Source: CAD feature listing. Evaluate the final solid. Frame: model axes, mm. A direction names the side the tool comes from. Round coordinates to 2 decimals unless told otherwise and drop trailing zeros. Loops run counter-clockwise (first coordinate to the right, second up) from the corner with the lowest first, then second, coordinate; pieces in that order, holes last. Notation, with made-up numbers: (49.25, 33.5) -> (105.25, 33.5) arc R23 ccw to (105.25, 52.5) -> close; hole circle Ø1 at (73, 71). An arc over 180 degrees is marked (long way). Write item = value, one per line.
from build123d import *

# Parameters (mm, degrees)
SKETCH_1_R          = 15.915
EXTRUDE_1_DEPTH     = 11
SKETCH_2_R          = 17
EXTRUDE_2_DEPTH     = 2
EXTRUDE_START       = 2
SKETCH_3_R          = 17
EXTRUDE_3_DEPTH     = 2
SKETCH_4_R          = 9.5
SKETCH_4_R_2        = 7.5
CUT_EXTRUDE_1_DEPTH = 0.5
SKETCH_4_3_R        = 7.5
SKETCH_4_3_R_2      = 5
CUT_EXTRUDE_2_DEPTH = 1.5
SKETCH_4_4_R        = 5
SKETCH_4_4_R_2      = 4
CUT_EXTRUDE_3_DEPTH = 0.5
SKETCH_4_5_R        = 4
CUT_EXTRUDE_4_DEPTH = 29.337254631
CUT_EXTRUDE_START   = -0.5
SKETCH_6_R          = 9.5
SKETCH_6_R_2        = 7.5
CUT_EXTRUDE_5_DEPTH = 0.5
CUT_EXTRUDE_START_2 = -1.5
SKETCH_6_3_R        = 7.5
SKETCH_6_3_R_2      = 5
CUT_EXTRUDE_6_DEPTH = 1.5
SKETCH_6_5_R        = 5
SKETCH_6_5_R_2      = 4
CUT_EXTRUDE_7_DEPTH = 0.5


with BuildPart() as part:
    # Sketch 1 → Extrude 1 (new body)
    with BuildSketch(Plane(origin=(0, 0, 0), x_dir=(1, 0, 0), z_dir=(0, 1, 0))):
        with Locations(Location((0, 0, 0), (0, 0, 270))):
            Circle(SKETCH_1_R)
    extrude(amount=EXTRUDE_1_DEPTH)

    # Sketch 2 → Extrude 2 (add)
    with BuildSketch(Plane(origin=(0, 11, 0), x_dir=(1, 0, 0), z_dir=(0, 1, 0))):
        with Locations(Location((0, 0, 0), (0, 0, 270))):
            Circle(SKETCH_2_R)
    extrude(amount=EXTRUDE_2_DEPTH)

    # Sketch 3 → Extrude 3 (add)
    with BuildSketch(Plane.XZ.offset(EXTRUDE_START)):
        with Locations(Location((0, 0, 0), (0, 0, 90))):
            Circle(SKETCH_3_R)
    extrude(amount=-EXTRUDE_3_DEPTH)

    # Sketch 4 → Cut-Extrude 1 (cut)
    with BuildSketch(Plane.XZ.offset(2)):
        with Locations(Location((0, 0, 0), (0, 0, 270))):
            Circle(SKETCH_4_R)
        with Locations(Location((0, 0, 0), (0, 0, 270))):
            Circle(SKETCH_4_R_2, mode=Mode.SUBTRACT)
    extrude(amount=-CUT_EXTRUDE_1_DEPTH, mode=Mode.SUBTRACT)

    # Sketch 4_3 → Cut-Extrude 2 (cut)
    with BuildSketch(Plane.XZ.offset(2)):
        with Locations(Location((0, 0, 0), (0, 0, 270))):
            Circle(SKETCH_4_3_R)
        with Locations(Location((0, 0, 0), (0, 0, 270))):
            Circle(SKETCH_4_3_R_2, mode=Mode.SUBTRACT)
    extrude(amount=-CUT_EXTRUDE_2_DEPTH, mode=Mode.SUBTRACT)

    # Sketch 4_4 → Cut-Extrude 3 (cut)
    with BuildSketch(Plane.XZ.offset(2)):
        with Locations(Location((0, 0, 0), (0, 0, 270))):
            Circle(SKETCH_4_4_R)
        with Locations(Location((0, 0, 0), (0, 0, 270))):
            Circle(SKETCH_4_4_R_2, mode=Mode.SUBTRACT)
    extrude(amount=-CUT_EXTRUDE_3_DEPTH, mode=Mode.SUBTRACT)

    # Sketch 4_5 → Cut-Extrude 4 (cut, through all)
    with BuildSketch(Plane.XZ.offset(2)):
        with Locations(Location((0, 0, 0), (0, 0, 270))):
            Circle(SKETCH_4_5_R)
    extrude(amount=-CUT_EXTRUDE_4_DEPTH, mode=Mode.SUBTRACT)

    # Sketch 6 → Cut-Extrude 5 (cut)
    with BuildSketch(Plane(origin=(0, 13, 0), x_dir=(1, 0, 0), z_dir=(0, 1, 0)).offset(CUT_EXTRUDE_START)):
        with Locations(Location((0, 0, 0), (0, 0, 90))):
            Circle(SKETCH_6_R)
        with Locations(Location((0, 0, 0), (0, 0, 90))):
            Circle(SKETCH_6_R_2, mode=Mode.SUBTRACT)
    extrude(amount=CUT_EXTRUDE_5_DEPTH, mode=Mode.SUBTRACT)

    # Sketch 6_3 → Cut-Extrude 6 (cut)
    with BuildSketch(Plane(origin=(0, 13, 0), x_dir=(1, 0, 0), z_dir=(0, 1, 0)).offset(CUT_EXTRUDE_START_2)):
        with Locations(Location((0, 0, 0), (0, 0, 90))):
            Circle(SKETCH_6_3_R)
        with Locations(Location((0, 0, 0), (0, 0, 90))):
            Circle(SKETCH_6_3_R_2, mode=Mode.SUBTRACT)
    extrude(amount=CUT_EXTRUDE_6_DEPTH, mode=Mode.SUBTRACT)

    # Sketch 6_5 → Cut-Extrude 7 (cut)
    with BuildSketch(Plane(origin=(0, 13, 0), x_dir=(1, 0, 0), z_dir=(0, 1, 0)).offset(CUT_EXTRUDE_START)):
        with Locations(Location((0, 0, 0), (0, 0, 270))):
            Circle(SKETCH_6_5_R)
        with Locations(Location((0, 0, 0), (0, 0, 90))):
            Circle(SKETCH_6_5_R_2, mode=Mode.SUBTRACT)
    extrude(amount=CUT_EXTRUDE_7_DEPTH, mode=Mode.SUBTRACT)


solid = part.part
1. Line query: probe 1 along X at (y, z) = (-1.3, 0); probe 2 along Y at (x, z) = (-13, -10); probe 3 along X at (y, z) = (11.75, 1.5). Output: solid intervals per line, ascending. Write a range as from..to.
Evaluation:
probe_1 = -17..-7.5, -5..-4, 4..5, 7.5..17
probe_2 = -2..0, 11..13
probe_3 = -16.93..-7.35, -4.77..-3.71, 3.71..4.77, 7.35..16.93
2. Section query A-A (y = 9.25). Return the cut outline in (x, z) (3 decimals).
Evaluation:
outline = circle Ø31.83 at (0, 0); hole circle Ø8 at (0, 0)
3. Section query C-C (z = 12). Return the cut outline in (x, y), then the cut area to 3 significant figures.
Evaluation:
outline = (-12.04, -2) -> (12.04, -2) -> (12.04, 0) -> (10.45, 0) -> (10.45, 11) -> (12.04, 11) -> (12.04, 13) -> (-12.04, 13) -> (-12.04, 11) -> (-10.45, 11) -> (-10.45, 0) -> (-12.04, 0) -> close
area = 326 mm²
4. Contact query for flat-ended pins moving along their axis: pin 1 Ø4 at (y, z) = (8.5, 5) entering from -X; pin 2 Ø11.5 at (x, z) = (0, 0) entering from -Y; pin 3 Ø2 at (x, y) = (-6, 0.5) entering from +Z; pin 4 Ø3 at (x, z) = (-0.5, 1.5) entering from +Y. Output: stop coordinate, or through.
Evaluation:
pin_1 = -15.63
pin_2 = -1.5
pin_3 = 16.21
pin_4 = through
5. Set-up query: faces 4 (the face through (4.88, 11.99, 1.08)), 5 (the face through (-13, 11, 10)), 6 (the face through (8, -1.5, -1)). Return all of +Z, -Z, +X, -X, +Y, -Y with unobstructed straight access to the full face (end or side cutting, diameter ignored); none if empty.
Evaluation:
face_4 = +Y
face_5 = none
face_6 = -Y
6. Section query B-B (x = -13). Return the cut outline in (y, z).
Evaluation:
outline = (-2, -10.95) -> (0, -10.95) -> (0, -9.18) -> (11, -9.18) -> (11, -10.95) -> (13, -10.95) -> (13, 10.95) -> (11, 10.95) -> (11, 9.18) -> (0, 9.18) -> (0, 10.95) -> (-2, 10.95) -> close
7. Mould query, pull axis Z, two halves, no side actions, for faces 1 (the face through (7, -2, 7)), 2 (the face through (-8, 12.5, -1)), 3 (the face through (4.78, 5.42, 15.18)). Classes: released by +Z, released by -Z, zero draft, split by the parting line, or undercut.
Evaluation:
face_1 = zero draft
face_2 = undercut
face_3 = split by the parting line
